Model file for the job. Use its own axes, mm. A direction names the side the tool comes from. Round coordinates to 2 decimals unless told otherwise and drop trailing zeros. Loops run counter-clockwise (first coordinate to the right, second up) from the corner with the lowest first, then second, coordinate; pieces in that order, holes last. Notation, with made-up numbers: (20, 78.5) - (53, 78.5) arc R17 cw to (53, 107.5) - close; hole circle Ø4 at (-34, -8). An arc over 180 degrees is marked (long way). Use one line per item in the form item = value.
from build123d import *

# Parameters (mm, degrees)
SKETCH2_W           = 50.8
SKETCH2_H           = 127
BOSS_EXTRUDE1_DEPTH = 6.35
SKETCH3_W           = 19.05
SKETCH3_H           = 6.35
BOSS_EXTRUDE2_DEPTH = 6.35
SKETCH5_W           = 50.8
SKETCH5_H           = 6.35
BOSS_EXTRUDE3_DEPTH = 6.35
SKETCH6_R           = 1.524
CUT_EXTRUDE1_DEPTH  = 143.839717866


with BuildPart() as part:
    # Sketch2 → Boss-Extrude1 (new body)
    with BuildSketch(Plane(origin=(0, 0, 0), x_dir=(0, 0, -1), z_dir=(1, 0, 0))):
        with Locations((25.4, 63.5)):
            Rectangle(SKETCH2_W, SKETCH2_H)
    extrude(amount=BOSS_EXTRUDE1_DEPTH)

    # Sketch3 → Boss-Extrude2 (add)
    with BuildSketch(Plane(origin=(6.35, 0, 0), x_dir=(0, 0, -1), z_dir=(1, 0, 0))):
        with Locations((25.4, -3.175)):
            Rectangle(SKETCH3_W, SKETCH3_H)
    extrude(amount=-BOSS_EXTRUDE2_DEPTH)

    # Sketch5 → Boss-Extrude3 (add)
    with BuildSketch(Plane.ZY):
        with Locations((-25.4, 130.175)):
            Rectangle(SKETCH5_W, SKETCH5_H)
    extrude(amount=-BOSS_EXTRUDE3_DEPTH)

    # Sketch6 → Cut-Extrude1 (cut, through all)
    with BuildSketch(Plane(origin=(6.35, 0, 0), x_dir=(0, 0, -1), z_dir=(1, 0, 0))):
        with Locations((25.4, 130.175)):
            Circle(SKETCH6_R)
    extrude(amount=-CUT_EXTRUDE1_DEPTH, mode=Mode.SUBTRACT)


solid = part.part
1. Cut at B-B, the plane x = 4.25. Give the cut face in (y, z) (3 decimals), plus the area to 3 significant figures.
Geometry check:
outline = (-6.35, -34.925) - (0, -34.925) - (0, -50.8) - (133.35, -50.8) - (133.35, 0) - (0, 0) - (0, -15.875) - (-6.35, -15.875) - close; hole circle Ø3.048 at (130.175, -25.4)
area = 6,890 mm^2
2. Wall check: probe 1 along Y at (x, z) = (3.5, -25.4); probe 2 along Y at (x, z) = (0.5, -45). Give the ranges that are in metal, low to high.
Geometry check:
probe_1 = -6.35 to 128.65, 131.7 to 133.35
probe_2 = 0 to 133.35
3. Flat gauge pins, fed straight in: pin 1 (1.9 mm diameter, centred on x = 2.5, z = -11, fed in from -Y); pin 2 (3 mm diameter, centred on x = 3, y = -4.5, fed in from +Z) (3 decimals); pin 3 (2.5 mm diameter, centred on y = 130.175, z = -25.4, fed in from +X); pin 4 (1.9 mm diameter, centred on x = 4.5, y = -2.5, fed in from -Z) (3 decimals). Where does each tip first touch, or does it go through?
Geometry check:
pin_1 = 0
pin_2 = -15.875
pin_3 = through
pin_4 = -34.925
4. Cut at C-C, the plane z = -4. Give the cut face in (x, y).
Geometry check:
outline = (0, 0) - (6.35, 0) - (6.35, 133.35) - (0, 133.35) - close
5. Tool access for faces 5 (the flat face through (3, -6.35, -25)), 6 (the flat face through (3, -3, -34.925)), 7 (the flat face through (3, 0, -8)): list every direction of +Z, -Z, +X, -X, +Y, -Y with a clear straight run to the whole face (end or side of a thin tool).
Geometry check:
face_5 = +Z, -Z, +X, -X, -Y
face_6 = -Z, +X, -X, -Y
face_7 = +Z, +X, -X, -Y
6. Pull direction Y, two halves, no side cores. Call faces 1 (the flat face through (3, -3, -15.875)), 2 (the flat face through (3, 0, -43)), 3 (the flat face through (3, 133.35, -26)), 4 (the cylindrical face through (3.219, 130.633, -26.854)): +Y half, -Y half, draft (parallel to the pull), parting line (faces both ways), or undercut.
Geometry check:
face_1 = draft
face_2 = -Y half
face_3 = +Y half
face_4 = undercut
7. Cut at A-A, the plane z = -25.4. Give the cut face in (x, y), plus the area to 3 significant figures.
Geometry check:
outline = (0, -6.35) - (6.35, -6.35) - (6.35, 128.65) - (0, 128.65) - close; (0, 131.7) - (6.35, 131.7) - (6.35, 133.35) - (0, 133.35) - close
area = 868 mm^2
